Job drawing, mm, ordinate dimensions from the low corner. One solid piece. A direction names the side the tool comes from. Round coordinates to 2 decimals unless told otherwise and drop trailing zeros. Loops run counter-clockwise (first coordinate to the right, second up) from the corner with the lowest first, then second, coordinate; pieces in that order, holes last.
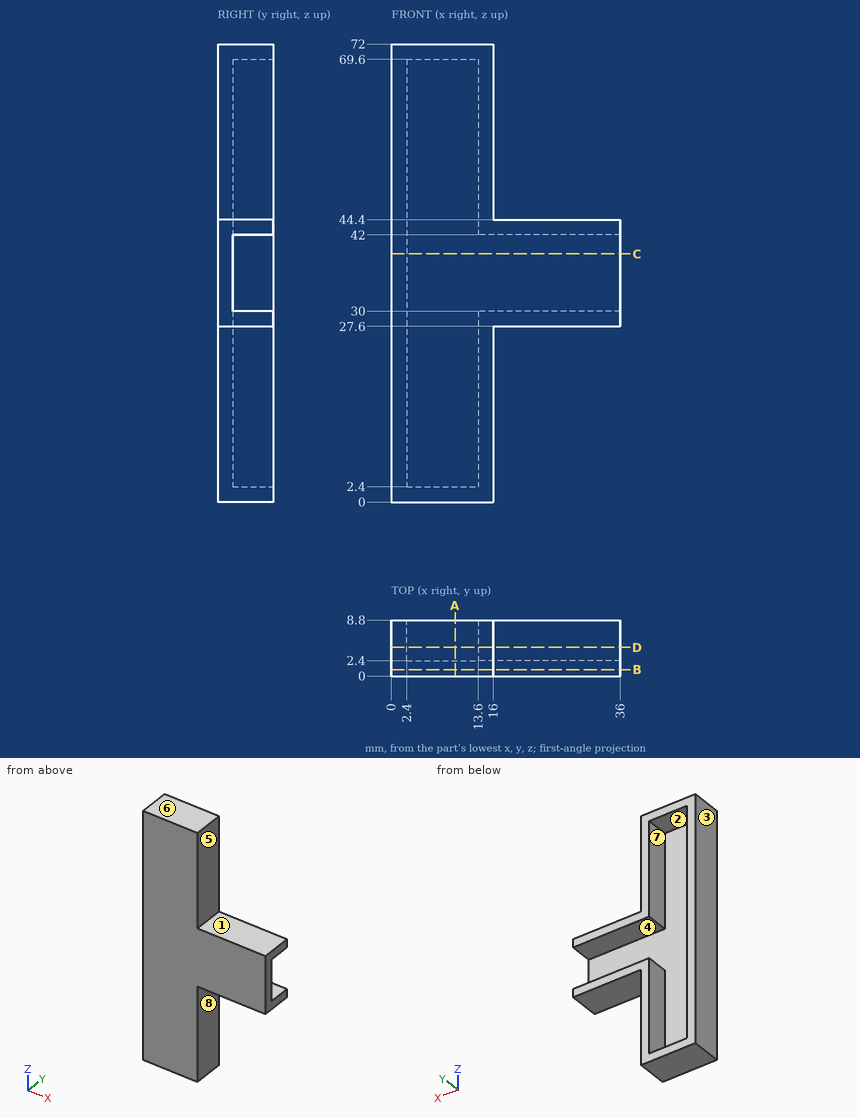
Item 1: 3-axis set-ups, long thin cutter, end or side, ignore diameter. For the marked faces 4, 5, 6, 7 and 8: which of +Z, -Z, +X, -X, +Y, -Y reach the whole face in a straight line?
Answers follow:
face 4: +X, +Y
face 5: +Z, +X, +Y, -Y
face 6: +Z, +X, -X, +Y, -Y
face 7: +Y
face 8: -Z, +X, +Y, -Y
Item 2: Cut at D-D, the plane y = 4.5. Give the cut face in (x, z).
Answers follow:
outline: (0, 0) - (16, 0) - (16, 27.6) - (36, 27.6) - (36, 30) - (13.6, 30) - (13.6, 2.4) - (2.4, 2.4) - (2.4, 69.6) - (13.6, 69.6) - (13.6, 42) - (36, 42) - (36, 44.4) - (16, 44.4) - (16, 72) - (0, 72) - close
Item 3: Cut at A-A, the plane x = 10. Give the cut face in (y, z).
Answers follow:
outline: (0, 0) - (8.8, 0) - (8.8, 2.4) - (2.4, 2.4) - (2.4, 69.6) - (8.8, 69.6) - (8.8, 72) - (0, 72) - close
Item 4: Two-plate mould, pull along Z, no slides. Class the marked faces 1, 2 and 3: released by +Z, released by -Z, zero draft, split by the parting line, or undercut.
Answers follow:
face 1: released by +Z
face 2: undercut
face 3: zero draft
Item 5: Flat gauge pins, fed straight in: P1, Ø4, axis at x = 25.5, z = 37, coming from the +Y side; P2, Ø4.5, axis at x = 26, y = 6, coming from the -Z side; P3, Ø4, axis at x = 5.5, y = 4.5, coming from the -Z side; P4, Ø1, axis at y = 2, z = 49, coming from the +X side. Where does each tip first touch, or does it go through?
Answers follow:
P1: stops at y = 2.4
P2: stops at z = 27.6
P3: stops at z = 0
P4: stops at x = 16
Item 6: Cut at C-C, the plane z = 39. Give the cut face in (x, y).
Answers follow:
outline: (0, 0) - (36, 0) - (36, 2.4) - (2.4, 2.4) - (2.4, 8.8) - (0, 8.8) - close
Item 7: Probe line 1 (Z direction, x = 30.5, y = 4); line 2 (Z direction, x = 5, y = 8.75); line 3 (X direction, y = 5.25, z = 50.5). List the from-to ranges inside material, lowest first.
Answers follow:
line 1: z = 27.6 to 30, 42 to 44.4
line 2: z = 0 to 2.4, 69.6 to 72
line 3: x = 0 to 2.4, 13.6 to 16
Item 8: Cut at B-B, the plane y = 1. Give the cut face in (x, z).
Answers follow:
outline: (0, 0) - (16, 0) - (16, 27.6) - (36, 27.6) - (36, 44.4) - (16, 44.4) - (16, 72) - (0, 72) - close
